Part model, mm, in its own coordinate system. Face numbers are marked on the shaded views. Give positions to 0.01 mm unless a question says otherwise; leave off trailing zeros. Write each loop counter-clockwise with the first axis right and the second up, starting at its lowest first coordinate (ties: lowest second). Pieces come first, ordered by that corner, then holes.
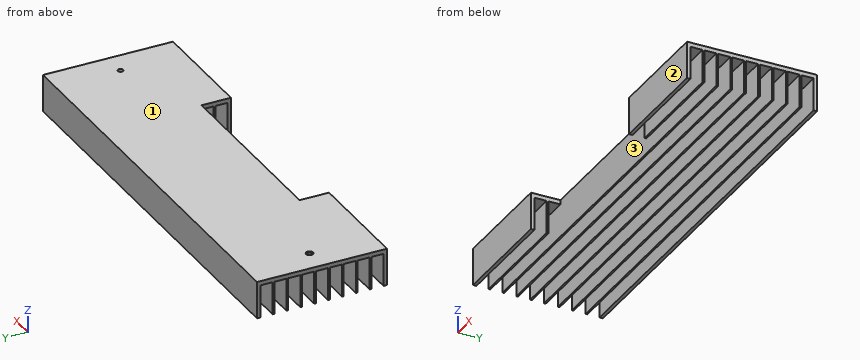
```python
from build123d import *

# Parameters (mm, degrees)
F0_W     = 1
F0_H     = 19
F0_W_2   = 2
F1_DEPTH = 120
F2_R     = 1.5
F3_DEPTH = 21.501
F4_SIZE  = 0.5
F5_W     = 110
F5_H     = 21.5
F6_DEPTH = 17


with BuildPart() as f1:
    # F0 (on Right) → F1 (new body, symmetric)
    with BuildSketch(Plane.YZ):
        with Locations((-4, 0)):
            Rectangle(F0_W, F0_H)
        with Locations((4, 0)):
            Rectangle(F0_W, F0_H)
        with Locations((-12, 0)):
            Rectangle(F0_W, F0_H)
        with Locations((-20, 0)):
            Rectangle(F0_W, F0_H)
        with Locations((12, 0)):
            Rectangle(F0_W, F0_H)
        with Locations((20, 0)):
            Rectangle(F0_W, F0_H)
        with Locations((28, 0)):
            Rectangle(F0_W, F0_H)
        with Locations((-28, 0)):
            Rectangle(F0_W, F0_H)
        with Locations((36.5, 0)):
            Rectangle(F0_W_2, F0_H)
        with Locations((-36.5, 0)):
            Rectangle(F0_W_2, F0_H)
        Polygon((-11.5, 9.5), (-4.5, 9.5), (-3.5, 9.5), (3.5, 9.5), (4.5, 9.5), (11.5, 9.5), (12.5, 9.5), (19.5, 9.5), (20.5, 9.5), (27.5, 9.5), (28.5, 9.5), (35.5, 9.5), (37.5, 9.5), (37.5, 12), (-37.5, 12), (-37.5, 9.5), (-35.5, 9.5), (-28.5, 9.5), (-27.5, 9.5), (-20.5, 9.5), (-19.5, 9.5), (-12.5, 9.5), align=None)
    extrude(amount=F1_DEPTH, both=True)

    # F2 (on face) → F3 (cut, through all)
    with BuildSketch(Plane.XY.offset(12)):
        with Locations((-106, 0)):
            Circle(F2_R)
        with Locations((106, 0)):
            Circle(F2_R)
    extrude(amount=-F3_DEPTH, mode=Mode.SUBTRACT)

    # F4
    f4_edges = [f1.edges().sort_by_distance(p)[0] for p in [
        (-107.5, 0, 12),
        (-104.5, 0, 10.75),
        (-107.5, 0, 9.5),
    ]]
    chamfer(f4_edges, length=F4_SIZE)

    # F5 (on face) → F6 (cut)
    with BuildSketch(Plane.XZ.offset(37.5)):
        with Locations((0, 1.25)):
            Rectangle(F5_W, F5_H)
    extrude(amount=-F6_DEPTH, mode=Mode.SUBTRACT)


solid = f1.part
```
1) Saw through at C-C, the plane z = -3.5. Count the separate pieces of the cut face and the enclosed holes in it, then the cut area to 3 significant figures.
Answers follow:
separate pieces: 12
enclosed holes: 0
area: 2,550 mm2
2) Pin check, flat tips, straight feed: pin 1 Ø1 at (x, z) = (-54, 8.5) entering from -Y; pin 2 Ø3.5 at (x, y) = (-103.5, -32) entering from -Z; pin 3 Ø2 at (y, z) = (1.5, 4.5) entering from +X. Stop position of each tip, or through.
Answers follow:
pin 1: stops at y = -20.5
pin 2: stops at z = 9.5
pin 3: passes through
3) Wall check: L1, parallel to Y at x = 106, z = 10.8; L2, parallel to Z at x = -104.5, y = 8. Give the ranges that are in metal, low to high.
Answers follow:
L1: y = -37.5 to -1.5, 1.5 to 37.5
L2: z = 9.5 to 12
4) Saw through at D-D, the plane y = 16. Write the cut outline in (x, z), then the cut area to 3 significant figures.
Answers follow:
outline: (-120, 9.5) - (120, 9.5) - (120, 12) - (-120, 12) - close
area: 600 mm2
5) Saw through at A-A, the plane y = -25. Write the cut outline in (x, z), then the cut area to 3 significant figures.
Answers follow:
outline: (-120, 9.5) - (-55, 9.5) - (-55, 12) - (-120, 12) - close; (55, 9.5) - (120, 9.5) - (120, 12) - (55, 12) - close
area: 325 mm2
6) Two-plate mould, pull along Y, no slides. Class the marked faces 1, 2 and 3: +Y half, -Y half, draft (parallel to the pull), parting line (faces both ways), or undercut.
Answers follow:
face 1: draft
face 2: -Y half
face 3: undercut
